Here's how the part is built. I have some questions about the finished solid (model axes, mm). Face numbers are marked on the shaded views. A direction names the side the tool comes from. Coordinates: 2 decimals unless noted, no trailing zeros. Loops run counter-clockwise (first coordinate to the right, second up) from the corner with the lowest first, then second, coordinate; pieces in that order, holes last.
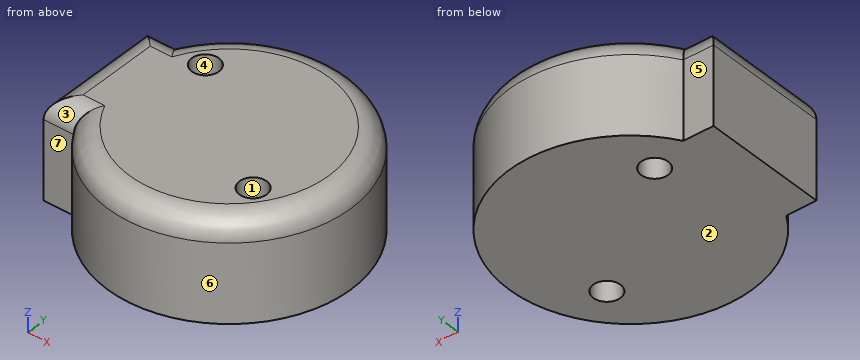
from build123d import *

# Parameters (mm, degrees)
SKETCH1_R           = 14.224
BOSS_EXTRUDE1_DEPTH = 11.684
SKETCH2_W           = 10.862447087
SKETCH2_H           = 14.605
BOSS_EXTRUDE2_DEPTH = 11.684
FILLET1_R           = 2.54
SKETCH3_R           = 1.5875
CUT_EXTRUDE1_DEPTH  = 11.684


with BuildPart() as part:
    # Sketch1 → Boss-Extrude1 (new body)
    with BuildSketch(Plane.XY):
        Circle(SKETCH1_R)
    extrude(amount=BOSS_EXTRUDE1_DEPTH)

    # Sketch2 → Boss-Extrude2 (add)
    with BuildSketch(Plane.XY.offset(11.684)):
        with Locations((-10.316776457, 0)):
            Rectangle(SKETCH2_W, SKETCH2_H)
    extrude(amount=-BOSS_EXTRUDE2_DEPTH)

    # Fillet1
    fillet1_edges = [part.edges().sort_by_distance(p)[0] for p in [
        (-13.97718912, 7.3025, 11.684),
        (-15.748, 0, 11.684),
        (-13.97718912, -7.3025, 11.684),
        (14.224, 0, 11.684),
    ]]
    fillet(fillet1_edges, radius=FILLET1_R - 0.0001)  # a hair under: the kernel refuses the full size

    # Sketch3 → Cut-Extrude1 (cut)
    with BuildSketch(Plane(origin=(0, 0, 0), x_dir=(-1, 0, 0), z_dir=(0, 0, -1))):
        with Locations((7.576884905, 5.772039513)):
            Circle(SKETCH3_R)
        with Locations((-7.576884905, -5.772039513)):
            Circle(SKETCH3_R)
    extrude(amount=-CUT_EXTRUDE1_DEPTH, mode=Mode.SUBTRACT)


solid = part.part
Q1. For the marked faces 5, 6 and 7, which set-ups out of +Z, -Z, +X, -X, +Y, -Y let a thin tool reach every point of the face, with its end or its side?
Q2. Will these pins go through, and if not, where does the flat tip stop? P1, Ø3, axis at x = -15, z = 6.5, coming from the -Y side; P2, Ø1.9, axis at x = 7.58, y = -5.77, coming from the -Z side; P3, Ø1.8, axis at x = -13.5, z = 6.5, coming from the +Y side; P4, Ø6, axis at x = -8.5, z = 5.5, coming from the -Y side.
Q3. Please list where these lines run through material, in increasing order: probe 1 along X at (y, z) = (-5.75, 4.75); probe 2 along Y at (x, z) = (-6.5, 9.5); probe 3 along Y at (x, z) = (-7.75, 9.5).
Q4. We'd pull the mould along Y, two halves only. Please class the marked faces 1, 2, 3 and 4: pulls with the +Y half, pulls with the -Y half, needs draft (parallel to the pull), parting line crosses it, or undercut.
Q5. Suppose I cut it at A-A on z = 4. Write out the boundary of the cut face in (x, y) (1 decimal).
Check values:
1. face 5: +Z, -Z, -X, +Y
1. face 6: +Z, -Z
1. face 7: +Z, -Z, -X, -Y
2. P1: stops at y = -7.3
2. P2: passes through
2. P3: stops at y = 7.3
2. P4: stops at y = -13.12
3. probe 1: x = -15.75 to 5.99, 9.16 to 13.01
3. probe 2: y = -12.62 to 4.61, 6.94 to 12.62
3. probe 3: y = -11.9 to 4.19, 7.35 to 11.9
4. face 1: undercut
4. face 2: needs draft
4. face 3: pulls with the -Y half
4. face 4: undercut
5. outline: (-15.7, -7.3) - (-12.2, -7.3) arc R14.2 ccw (long way) to (-12.2, 7.3) - (-15.7, 7.3) - close; hole circle Ø3.2 at (-7.6, 5.8); hole circle Ø3.2 at (7.6, -5.8)
